The listing builds one solid part. Answer for the finished solid, in the listing's coordinates (mm). Face numbers are marked on the shaded views. A direction names the side the tool comes from. Coordinates: 2 decimals unless noted, no trailing zeros. Loops run counter-clockwise (first coordinate to the right, second up) from the corner with the lowest first, then second, coordinate; pieces in that order, holes last. Notation, with made-up numbers: (-2, 19) - (6, 19) arc R25 ccw to (6, 38) - close; hole circle Ø5 at (-20, 81). An arc over 180 degrees is marked (long way). One line per question, with ' | ' between items.
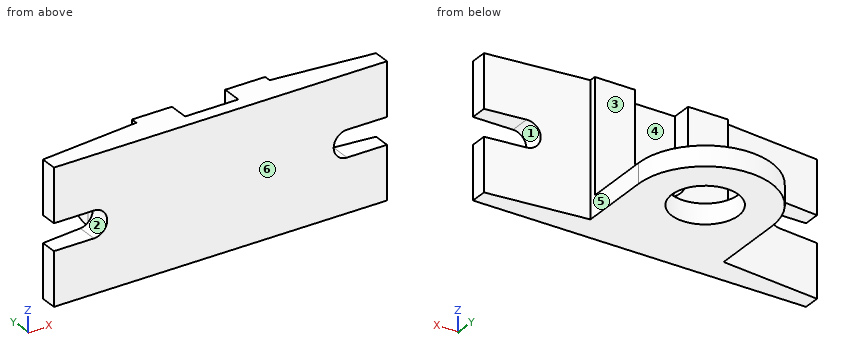
from build123d import *

# Parameters (mm, degrees)
BOSS_EXTRUDE1_DEPTH = 200
CUT_EXTRUDE1_DEPTH  = 30
CUT_EXTRUDE2_DEPTH  = 325.03703492
SKETCH5_R           = 50
BOSS_EXTRUDE2_DEPTH = 30


with BuildPart() as part:
    # Sketch2 → Boss-Extrude1 (new body)
    with BuildSketch(Plane.XY):
        Polygon((-250, 0), (250, 0), (250, 25), (100, 40), (100, 50), (-100, 50), (-100, 40), (-250, 25), align=None)
    extrude(amount=-BOSS_EXTRUDE1_DEPTH)

    # Sketch3 → Cut-Extrude1 (cut)
    with BuildSketch(Plane(origin=(0, 50, 0), x_dir=(1, 0, 0), z_dir=(0, 1, 0))):
        with BuildLine():
            Line((-40, 100), (-40, 0))
            Line((-40, 0), (40, 0))
            Line((40, 0), (40, 100))
            ThreePointArc((40, 100), (0, 140), (-40, 100))
        make_face()
    extrude(amount=-CUT_EXTRUDE1_DEPTH, mode=Mode.SUBTRACT)

    # Sketch4 → Cut-Extrude2 (cut, through all)
    with BuildSketch(Plane.XZ):
        with BuildLine():
            Line((-190, -80), (-250, -80))
            Line((-250, -80), (-250, -120))
            Line((-250, -120), (-190, -120))
            ThreePointArc((-190, -120), (-170, -100), (-190, -80))
        make_face()
        with BuildLine():
            Line((250, -120), (250, -80))
            Line((250, -80), (190, -80))
            ThreePointArc((190, -80), (170, -100), (190, -120))
            Line((190, -120), (250, -120))
        make_face()
    extrude(amount=-CUT_EXTRUDE2_DEPTH, mode=Mode.SUBTRACT)

    # Sketch5 → Boss-Extrude2 (add)
    with BuildSketch(Plane(origin=(0, 0, -200), x_dir=(-1, 0, 0), z_dir=(0, 0, -1))):
        with BuildLine():
            Line((-100, 50), (-100, 150))
            ThreePointArc((-100, 150), (0, 250), (100, 150))
            Line((100, 150), (100, 50))
            Line((100, 50), (-100, 50))
        make_face()
        with Locations((0, 150)):
            Circle(SKETCH5_R, mode=Mode.SUBTRACT)
    extrude(amount=-BOSS_EXTRUDE2_DEPTH)


solid = part.part
Item 1: Find the intervals of material crossed by line 1 (Y direction, x = 0, z = -179); line 2 (Z direction, x = 17.5, y = 73); line 3 (Y direction, x = -71, z = -121.5), in increasing order. Write a range as [from, to].
Taken from the geometry:
line 1: y = [0, 100], [200, 250] | line 2: z = [-200, -170] | line 3: y = [0, 50]
Item 2: Find section C-C, the plane y = 118.5. Write down the section's boundary in (x, z), plus the area to 3 significant figures.
Taken from the geometry:
outline: (-100, -200) - (-38.83, -200) - (-38.83, -170) - (-100, -170) - close; (38.83, -200) - (100, -200) - (100, -170) - (38.83, -170) - close | area: 3,670 mm2
Item 3: Find section D-D, the plane z = -88. Write down the section's boundary in (x, y).
Taken from the geometry:
outline: (-174, 0) - (174, 0) - (174, 32.6) - (100, 40) - (100, 50) - (40, 50) - (40, 20) - (-40, 20) - (-40, 50) - (-100, 50) - (-100, 40) - (-174, 32.6) - close
Item 4: Each of these flat-tipped pins is pushed along its axis until it touches: pin 1 Ø9.5 at (x, y) = (207.5, 12) entering from +Z; pin 2 Ø8 at (y, z) = (49.5, -50.5) entering from -X; pin 3 Ø12 at (x, y) = (36, 180) entering from +Z; pin 4 Ø3 at (x, z) = (47.5, -67) entering from +Y. Where does it stop, or does it pass through?
Taken from the geometry:
pin 1: stops at z = 0 | pin 2: stops at x = -100 | pin 3: stops at z = -170 | pin 4: stops at y = 50
Item 5: Find section A-A, the plane x = -216. Write down the section's boundary in (y, z).
Taken from the geometry:
outline: (0, -200) - (28.4, -200) - (28.4, -120) - (0, -120) - close; (0, -80) - (28.4, -80) - (28.4, 0) - (0, 0) - close
Item 6: Find section B-B, the plane z = -150. Write down the section's boundary in (x, y).
Taken from the geometry:
outline: (-250, 0) - (250, 0) - (250, 25) - (100, 40) - (100, 50) - (-100, 50) - (-100, 40) - (-250, 25) - close
Item 7: The mould has two halves that part along X. Classify the marked faces 1, 2, 3 and 4: pulls with the +X half, pulls with the -X half, needs draft (parallel to the pull), parting line crosses it, or undercut.
Taken from the geometry:
face 1: pulls with the +X half | face 2: pulls with the -X half | face 3: needs draft | face 4: undercut
Item 8: Which of the six approach directions +Z, -Z, +X, -X, +Y, -Y give full straight-line access (tool end or side, diameter ignored) to the marked faces 5 and 6?
Taken from the geometry:
face 5: +Z, -Z, +X, +Y | face 6: +Z, -Z, +X, -X, -Y
